Verification items for the finished model (mm, model axes). Face numbers are marked on the shaded views. A direction names the side the tool comes from. Round coordinates to 2 decimals unless told otherwise and drop trailing zeros. Order: outer loops, then holes, each group sorted by start corner. A loop starts at its lowest first (then second) coordinate and runs counter-clockwise, first axis right, second up. Notation, with made-up numbers: M 52.5,33 L 56.5,33 A19 cw 56.5,62 Z; hole C 42.25,85 d11. An arc over 180 degrees is marked long. Return JSON: item names as keys, results as strings. Group by question number.
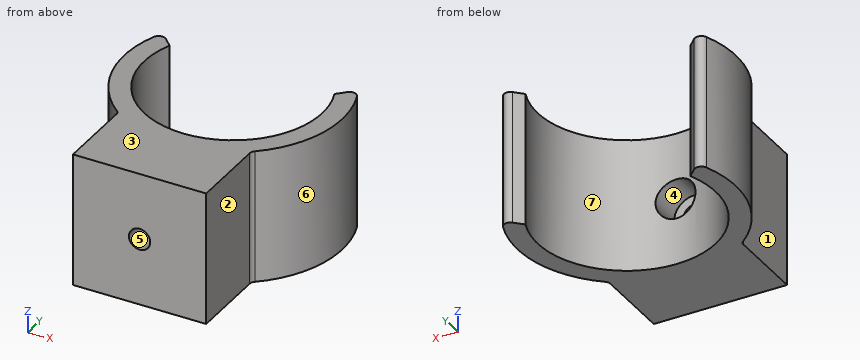
from build123d import *

# Parameters (mm, degrees)
CYLINDER_R     = 3
CYLINDER_DEPTH = 10
PAD_DEPTH      = 20
PAD001_DEPTH   = 20
SKETCH002_R    = 1.6
POCKET_DEPTH   = 32.268643
FILLET_R       = 1
FILLET001_R    = 1


with BuildPart() as cylinder:
    # Cylinder → Cylinder (new body)
    with BuildSketch(Plane(origin=(0, -18, 10), x_dir=(0, 0, 1), z_dir=(0, 1, 0))):
        Circle(CYLINDER_R)
    extrude(amount=CYLINDER_DEPTH)


with BuildPart() as fillet001:
    # Sketch → Pad (new body)
    with BuildSketch(Plane.XY):
        with BuildLine():
            ThreePointArc((-12.378308, 5), (0, -13.35), (12.378308, 5))
            Line((14.645951, 7.267643), (12.378308, 5))
            ThreePointArc((-14.645951, 7.267643), (0, -16.35), (14.645951, 7.267643))
            Line((-14.645951, 7.267643), (-12.378308, 5))
        make_face()
    extrude(amount=PAD_DEPTH)

    # Sketch001 → Pad001 (new body)
    with BuildSketch(Plane.XY.offset(20)):
        with BuildLine():
            ThreePointArc((-10, -10), (0, -14.142136), (10, -10))
            Line((10, -10), (10, -25))
            Line((10, -25), (-10, -25))
            Line((-10, -25), (-10, -10))
        make_face()
    extrude(amount=-PAD001_DEPTH)

    # Sketch002 → Pocket (cut, through all)
    with BuildSketch(Plane.XZ.offset(25)):
        with Locations((0, 10)):
            Circle(SKETCH002_R)
    extrude(amount=-POCKET_DEPTH, mode=Mode.SUBTRACT)

    # Cut: cut Cylinder
    add(cylinder.part, mode=Mode.SUBTRACT)

    # Fillet
    fillet_edges = [fillet001.edges().sort_by_distance(p)[0] for p in [
        (-14.645951, 7.267643, 10),
        (14.645951, 7.267643, 10),
    ]]
    fillet(fillet_edges, radius=FILLET_R)

    # Fillet001
    fillet001_edges = [fillet001.edges().sort_by_distance(p)[0] for p in [
        (-10, -12.93532, 10),
        (10, -12.93532, 10),
    ]]
    fillet(fillet001_edges, radius=FILLET001_R)


solid = fillet001.part
1. Access from +Z, -Z, +X, -X, +Y, -Y to the whole of each face (thin tool, end or side, straight path). Record for the marked faces 1, 2, 3 and 4.
2. Cross-section at C-C (z = 10). Enter the section's corners in (x, y), plus the area to 3 significant figures.
3. Go/stop test with flat-tipped pins: pin 1 (9.5 mm diameter, centred on y = -20, z = 8.5, fed in from -X); pin 2 (6 mm diameter, centred on x = 8, y = -4, fed in from -Z); pin 3 (8 mm diameter, centred on y = -8, z = 14.5, fed in from +X); pin 4 (7 mm diameter, centred on x = 0, z = 10, fed in from +Y). Record where each tip stops, or that it passes through.
4. Thickness scan on line 1 along Z through (x, y) = (0, -22.5); line 2 along Z through (x, y) = (0, -15.7); line 3 along X through (y, z) = (-8, 18.5). Record the ranges inside material, lowest first. Write a range as from..to.
5. Cross-section at D-D (y = -19.5). Enter the section's corners in (x, z), plus the area to 3 significant figures.
6. Cross-section at A-A (y = 0). Enter the section's corners in (x, z), plus the area to 3 significant figures.
7. Draft check along Y on the marked faces 5, 6 and 7. Enter one of: +Y half, -Y half, draft (parallel to the pull), parting line (faces both ways), or undercut.
8. Cross-section at B-B (x = 0). Enter the section's corners in (y, z).
Computed:
{
 "1": {"face 1": "+Z, -Z, -X, -Y", "face 2": "+Z, -Z, +X, -Y", "face 3": "+Z, +X, -X, +Y, -Y", "face 4": "+Y"},
 "2": {"outline": "M -15.25,5.89 A16.35 ccw -10.37,-12.64 A1 cw -10,-13.42 L -10,-25 L -1.6,-25 L -1.6,-18 L -3,-18 L -3,-13.01 A13.35 cw -12.38,5 L -13.61,6.23 A1 ccw Z; M 1.6,-25 L 10,-25 L 10,-13.42 A1 cw 10.37,-12.64 A16.35 ccw 15.25,5.89 A1 ccw 13.61,6.23 L 12.38,5 A13.35 cw 3,-13.01 L 3,-18 L 1.6,-18 Z", "area": "321 mm²"},
 "3": {"pin 1": "stops at x = -10", "pin 2": "passes through", "pin 3": "stops at x = 15.85", "pin 4": "stops at y = -12.88"},
 "4": {"line 1": "z = 0..8.4, 11.6..20", "line 2": "z = 0..7, 13..20", "line 3": "x = -14.26..-10.69, 10.69..14.26"},
 "5": {"outline": "M -10,0 L 10,0 L 10,20 L -10,20 Z; hole C 0,10 d3.2", "area": "392 mm²"},
 "6": {"outline": "M -16.35,0 L -13.35,0 L -13.35,20 L -16.35,20 Z; M 13.35,0 L 16.35,0 L 16.35,20 L 13.35,20 Z", "area": "120 mm²"},
 "7": {"face 5": "draft", "face 6": "parting line", "face 7": "undercut"},
 "8": {"outline": "M -25,0 L -13.35,0 L -13.35,7 L -18,7 L -18,8.4 L -25,8.4 Z; M -25,11.6 L -18,11.6 L -18,13 L -13.35,13 L -13.35,20 L -25,20 Z"}
}
